```python
from build123d import *

# Parameters (mm, degrees)
F1_DEPTH  = 27.94
F2_W      = 16.4592
F2_H      = 12.2074130923
F3_DEPTH  = 57.9374
F5_DEPTH  = 2.032
F6_DEPTH  = 25.4
F7_W      = 31.1324808757
F7_H      = 15.748
F8_DEPTH  = 25.4
F9_W      = 17.78
F9_H      = 31.1324808757
F10_DEPTH = 42.926


with BuildPart() as f1:
    # F0 (on Top) → F1 (new body)
    with BuildSketch(Plane.XY):
        with BuildLine():
            Line((-2.2859999444, 39.37), (-2.2859999444, 1.27))
            ThreePointArc((-2.2859999444, 1.27), (-1.2444716746, -1.2444716746), (1.27, -2.2859999444))
            Line((1.27, -2.2859999444), (21.59, -2.2859999444))
            ThreePointArc((21.59, -2.2859999444), (24.1044716746, -1.2444716746), (25.1459999444, 1.27))
            Line((25.1459999444, 1.27), (25.1459999444, 39.37))
            ThreePointArc((25.1459999444, 39.37), (24.1044716746, 41.8844716746), (21.59, 42.9259999444))
            Line((21.59, 42.9259999444), (1.27, 42.9259999444))
            ThreePointArc((1.27, 42.9259999444), (-1.2444716746, 41.8844716746), (-2.2859999444, 39.37))
        make_face()
        with BuildLine():
            Line((21.59, 0), (1.27, 0))
            ThreePointArc((1.27, 0), (0.3719743879, 0.3719743879), (0, 1.27))
            Line((0, 1.27), (0, 39.37))
            ThreePointArc((0, 39.37), (0.3719743879, 40.2680256121), (1.27, 40.64))
            Line((1.27, 40.64), (21.59, 40.64))
            ThreePointArc((21.59, 40.64), (22.4880256121, 40.2680256121), (22.86, 39.37))
            Line((22.86, 39.37), (22.86, 1.27))
            ThreePointArc((22.86, 1.27), (22.4880256121, 0.3719743879), (21.59, 0))
        make_face(mode=Mode.SUBTRACT)
    extrude(amount=F1_DEPTH)

    # F2 (on face) → F3 (cut)
    with BuildSketch(Plane.XZ.offset(2.2859999444)):
        with Locations((11.43, 19.8580278084)):
            Rectangle(F2_W, F2_H)
    extrude(amount=-F3_DEPTH, mode=Mode.SUBTRACT)

    # F4 (on Top) → F5 (join)
    with BuildSketch(Plane.XY):
        with BuildLine():
            Line((1.0258011753, 42.9636910558), (-3.6540816908, 42.9636910558))
            ThreePointArc((-3.6540816908, 42.9636910558), (-4.5256185939, 41.2599738136), (-4.8259983516, 39.37))
            Line((-4.8259983516, 39.37), (-4.8259983516, 1.27))
            ThreePointArc((-4.8259983516, 1.27), (-3.0405217725, -3.0405217725), (1.27, -4.8259983516))
            Line((1.27, -4.8259983516), (21.59, -4.8259983516))
            ThreePointArc((21.59, -4.8259983516), (25.9005217725, -3.0405217725), (27.6859983516, 1.27))
            Line((27.6859983516, 1.27), (27.6859983516, 39.37))
            ThreePointArc((27.6859983516, 39.37), (27.3856185939, 41.2599738136), (26.5140816908, 42.9636910558))
            Line((26.5140816908, 42.9636910558), (1.0258011753, 42.9636910558))
        make_face()
    extrude(amount=F5_DEPTH)

    # F6 (cut): a face of the model
    f6_faces = [f1.faces().sort_by_distance(p)[0] for p in [
        (11.43, 20.32, 2.032),
    ]]
    extrude(f6_faces, amount=-F6_DEPTH, mode=Mode.SUBTRACT)

    # F7 (on face) → F8 (join)
    with BuildSketch(Plane(origin=(-2.2859999444, 0, 0), x_dir=(0, -1, 0), z_dir=(-1, 0, 0))):
        with Locations((-19.8064594535, 20.066)):
            Rectangle(F7_W, F7_H)
    extrude(amount=-F8_DEPTH)

    # F9 (on face) → F10 (cut)
    with BuildSketch(Plane.XY.offset(27.94)):
        with Locations((11.4274583516, 19.8064594535)):
            Rectangle(F9_W, F9_H)
    extrude(amount=-F10_DEPTH, mode=Mode.SUBTRACT)


solid = f1.part
```
Geometry: final body of the model. Coordinates: model frame, mm. A direction names the side the tool comes from. Coordinates: 2 decimals unless noted, no trailing zeros. Order: outer loops, then holes, each group sorted by start corner. A loop starts at its lowest first (then second) coordinate and runs counter-clockwise, first axis right, second up. Notation, with made-up numbers: M -28.5,-36 L 22.5,-36 A18 ccw 22.5,-3 Z; hole C 81.5,31 d6. An arc over 180 degrees is marked long. Answer as CSV lines item,"result".
Q1. First-contact query: P1, Ø2.5, axis at y = 42, z = 18, coming from the -X side; P2, Ø1, axis at x = 22.5, z = 20.5, coming from the -Y side; P3, Ø4, axis at y = 37, z = 9, coming from the +X side. Flat tips, straight axial feed; report the tip coordinate or a pass-through.
Answers:
P1,"stops at x = -2.01"
P2,"stops at y = -2.26"
P3,"stops at x = 25.15"
Q2. Set-up query: faces 4 (the flat face through (12, 42.964, 1)), 5 (the flat face through (1, 20, 12.192)), 6 (the cylindrical face through (0.382, 0.362, 14.166)), 7 (the flat face through (11, 42, 25.962)), 8 (the flat face through (25.146, 20, 15)). Return all of +Z, -Z, +X, -X, +Y, -Y with unobstructed straight access to the full face (end or side cutting, diameter ignored); none if empty.
Answers:
face 4,"+Z, -Z, +X, -X, +Y"
face 5,"-Z"
face 6,"+Z, -Z"
face 7,"+Y, -Y"
face 8,"+Z, +X, +Y, -Y"
Q3. Line query: probe 1 along X at (y, z) = (12, 10.25); probe 2 along Y at (x, z) = (21, 7); probe 3 along Z at (x, y) = (8.5, 41). Output: solid intervals per line, ascending. Write a range as [from, to].
Answers:
probe 1,"x = [-2.29, 0], [22.86, 25.15]"
probe 2,"y = [-2.29, 0], [40.64, 42.93]"
probe 3,"z = [0, 13.75], [25.96, 27.94]"
Q4. Section D-D on z = 12.75. Return the cut outline in (x, y), and give its area (3 significant figures).
Answers:
outline,"M -2.29,1.27 A3.56 ccw 1.27,-2.29 L 21.59,-2.29 A3.56 ccw 25.15,1.27 L 25.15,39.37 A3.56 ccw 21.59,42.93 L 1.27,42.93 A3.56 ccw -2.29,39.37 Z; hole M 0,1.27 A1.27 ccw 1.27,0 L 21.59,0 A1.27 ccw 22.86,1.27 L 22.86,4.24 L 20.32,4.24 L 20.32,35.37 L 22.86,35.37 L 22.86,39.37 A1.27 ccw 21.59,40.64 L 1.27,40.64 A1.27 ccw 0,39.37 L 0,35.37 L 2.54,35.37 L 2.54,4.24 L 0,4.24 Z"
area,"460 mm^2"
Q5. Section B-B on x = 21. Count the separate pieces of the cut face and the enclosed holes in it, and give its area (3 significant figures).
Answers:
separate pieces,"3"
enclosed holes,"0"
area,"623 mm^2"
Q6. Section A-A on y = 12. Return the cut outline in (x, z).
Answers:
outline,"M -4.83,0 L 0,0 L 0,12.19 L 2.54,12.19 L 2.54,27.94 L -2.29,27.94 L -2.29,2.03 L -4.83,2.03 Z; M 20.32,12.19 L 22.86,12.19 L 22.86,0 L 27.69,0 L 27.69,2.03 L 25.15,2.03 L 25.15,27.94 L 20.32,27.94 Z"
Q7. Draft query along Y for faces 1 (the flat face through (19.66, 42, 20)), 2 (the flat face through (0, 20, 8)), 3 (the cylindrical face through (24.08, -1.27, 14.8)). Return one class per face: pulls with the +Y half, pulls with the -Y half, needs draft (parallel to the pull), parting line crosses it, or undercut.
Answers:
face 1,"needs draft"
face 2,"undercut"
face 3,"pulls with the -Y half"
